Geometry check sheet. Reference: drawing and pictorial views, mm from the part's lowest x, y, z. A direction names the side the tool comes from. Coordinates: 2 decimals unless noted, no trailing zeros. Loops run counter-clockwise (first coordinate to the right, second up) from the corner with the lowest first, then second, coordinate; pieces in that order, holes last. Notation, with made-up numbers: (28, -30) - (39, -30) arc R10 ccw to (39, -21) - close; hole circle Ø3 at (88.25, 78.25). An arc over 180 degrees is marked (long way). Write each question's results on one line, items separated by ' | '. Start each with the question number.
1. Gauge pin test, flat ends, axial feed: P1, Ø8.5, axis at x = 26.5, y = 48.5, coming from the -Z side; P2, Ø4, axis at y = 14.5, z = 48.5, coming from the -X side; P3, Ø4, axis at y = 30.5, z = 15, coming from the +X side. Record the tip position at first contact, or that the pin passes through.
2. Draft check along X on the marked faces 1 and 2. Enter one of: released by +X, released by -X, zero draft, split by the parting line, or undercut.
3. Tool access check on the marked faces 3 and 4. Record the directions out of +Z, -Z, +X, -X, +Y, -Y that give a thin tool (end or side, any length) a straight path to the whole face; none if there is none.
4. Cross-section at A-A (x = 23.5). Record the cut outline in (y, z).
5. Cross-section at B-B (y = 108.5). Record the cut outline in (x, z) (1 decimal).
6. Cross-section at C-C (z = 11.5). Give the number of separate pieces and of enclosed holes in the cut face, and give its area (3 significant figures).
7. Thickness scan on line 1 (X direction, y = 52, z = 18) (1 decimal); line 2 (Y direction, x = 66, z = 18.5) (1 decimal); line 3 (Y direction, x = 28, z = 33) (1 decimal). Record the ranges inside material, lowest first. Write a range as [from, to].
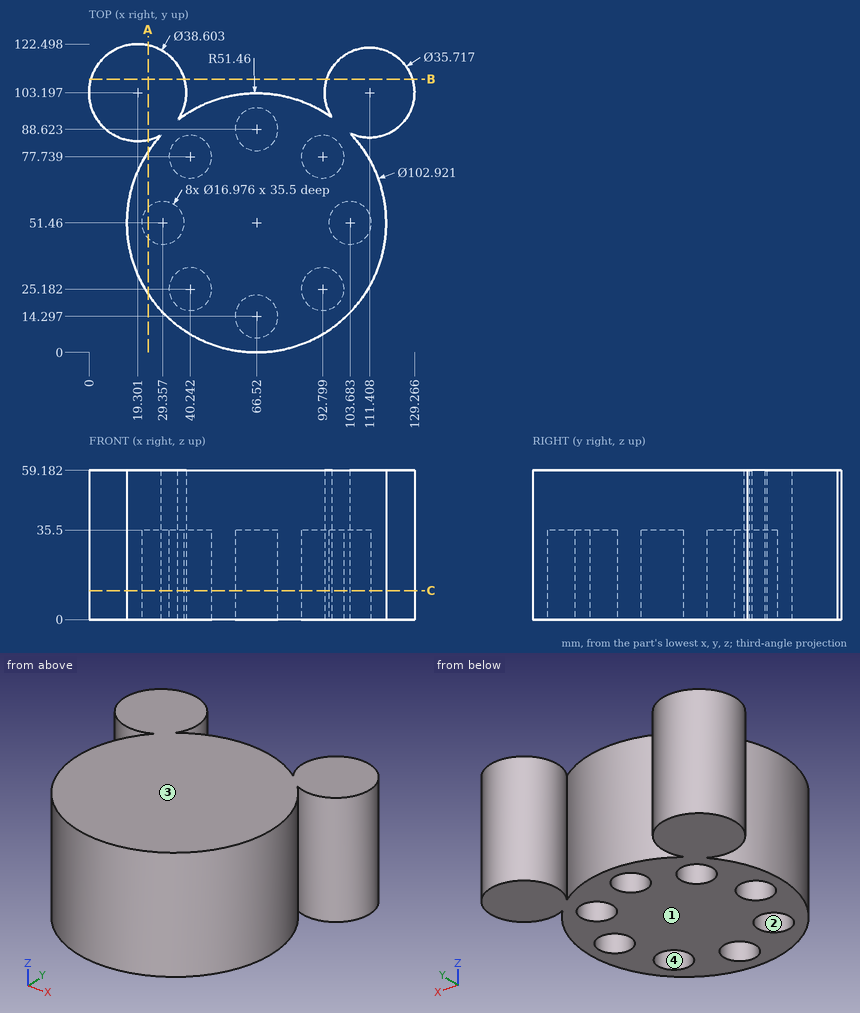
Established:
1) P1: z = 35.5 | P2: x = 28.76 | P3: x = 114.36
2) face 1: zero draft | face 2: undercut
3) face 3: +Z, +X, -X, +Y, -Y | face 4: -Z
4) outline: (23.22, 0) - (45.32, 0) - (45.32, 35.5) - (57.6, 35.5) - (57.6, 0) - (79.7, 0) - (79.7, 59.18) - (23.22, 59.18) - close; (84.36, 0) - (122.04, 0) - (122.04, 59.18) - (84.36, 59.18) - close
5) outline: (0.7, 0) - (37.9, 0) - (37.9, 59.2) - (0.7, 59.2) - close; (94.4, 0) - (128.5, 0) - (128.5, 59.2) - (94.4, 59.2) - close
6) separate pieces: 1 | enclosed holes: 8 | area: 8,670 mm^2
7) line 1: [15.1, 20.9], [37.8, 95.2], [112.2, 118] | line 2: [0, 5.8], [22.8, 80.2], [97.1, 102.9] | line 3: [17.3, 43.1], [59.8, 85.6], [86, 120.4]
